Geometry check sheet. Reference: drawing and pictorial views, mm from the part's lowest x, y, z. A direction names the side the tool comes from. Coordinates: 2 decimals unless noted, no trailing zeros. Write each loop counter-clockwise with the first axis right and the second up, starting at its lowest first coordinate (ties: lowest second). Pieces come first, ordered by that corner, then holes. Notation, with made-up numbers: (-12, 54) -> (-3, 54) arc R10 ccw to (-3, 62) -> close; hole circle Ø8 at (19.25, -35.5). An arc over 180 degrees is marked (long way). Use a Markdown table: item, result.
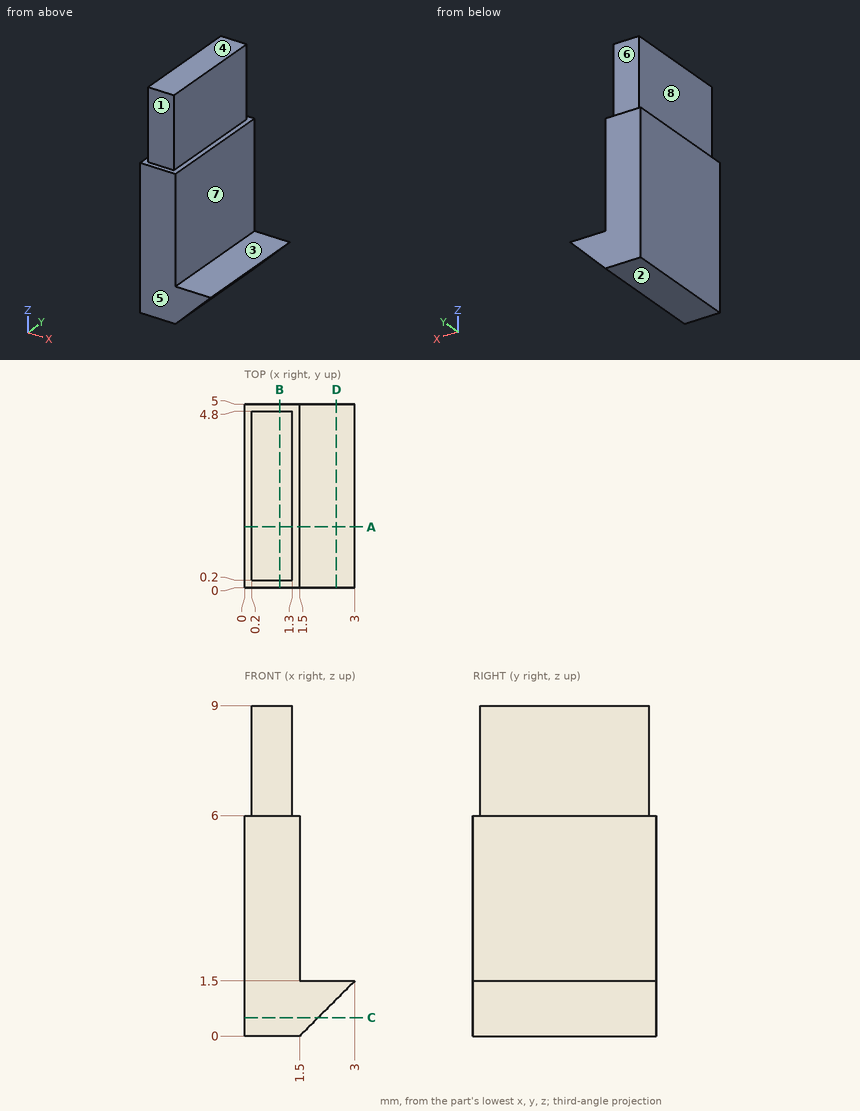
Item 1: Section check B-B on x = 0.95. Record the boundary of the cut face in (y, z).
Answer block:
| item | result |
|---|---|
| outline | (0, 0) -> (5, 0) -> (5, 6) -> (4.8, 6) -> (4.8, 9) -> (0.2, 9) -> (0.2, 6) -> (0, 6) -> close |
Item 2: Section check A-A on y = 1.65. Record the boundary of the cut face in (x, z).
Answer block:
| item | result |
|---|---|
| outline | (0, 0) -> (1.5, 0) -> (3, 1.5) -> (1.5, 1.5) -> (1.5, 6) -> (1.3, 6) -> (1.3, 9) -> (0.2, 9) -> (0.2, 6) -> (0, 6) -> close |
Item 3: Depth check by flat-ended pin: P1, Ø1.5, axis at x = 2.5, y = 1, coming from the -Z side; P2, Ø0.9, axis at x = 0.5, z = 7.5, coming from the +Y side; P3, Ø0.6, axis at x = 0.5, z = 7.5, coming from the -Y side; P4, Ø1, axis at x = 1.5, y = 2, coming from the +Z side. Enter the tip coordinate at first touch or a pass-through.
Answer block:
| item | result |
|---|---|
| P1 | stops at z = 0.25 |
| P2 | stops at y = 4.8 |
| P3 | stops at y = 0.2 |
| P4 | stops at z = 9 |
Item 4: Section check C-C on z = 0.5. Record the boundary of the cut face in (x, y), then the cut area to 3 significant figures.
Answer block:
| item | result |
|---|---|
| outline | (0, 0) -> (2, 0) -> (2, 5) -> (0, 5) -> close |
| area | 10.0 mm^2 |
Item 5: Tool access check on the marked faces 4, 5, 6, 7 and 8. Record the directions out of +Z, -Z, +X, -X, +Y, -Y that give a thin tool (end or side, any length) a straight path to the whole face; none if there is none.
Answer block:
| item | result |
|---|---|
| face 4 | +Z, +X, -X, +Y, -Y |
| face 5 | +Z, -Z, +X, -X, -Y |
| face 6 | +Z, +X, -X, +Y |
| face 7 | +Z, +X, +Y, -Y |
| face 8 | +Z, -X, +Y, -Y |
Item 6: Section check D-D on x = 2.5. Record the boundary of the cut face in (y, z).
Answer block:
| item | result |
|---|---|
| outline | (0, 1) -> (5, 1) -> (5, 1.5) -> (0, 1.5) -> close |
Item 7: Mould release check, pull along Z, two halves, no side actions. Record for the marked faces 1, 2 and 3: +Z half, -Z half, draft (parallel to the pull), parting line (faces both ways), or undercut.
Answer block:
| item | result |
|---|---|
| face 1 | draft |
| face 2 | -Z half |
| face 3 | +Z half |
Item 8: Thickness scan on L1, parallel to Y at x = 1, z = 8; L2, parallel to Z at x = 1.7, y = 1.8; L3, parallel to X at y = 2.25, z = 7.5. Record the ranges inside material, lowest first. Write a range as [from, to].
Answer block:
| item | result |
|---|---|
| L1 | y = [0.2, 4.8] |
| L2 | z = [0.2, 1.5] |
| L3 | x = [0.2, 1.3] |
